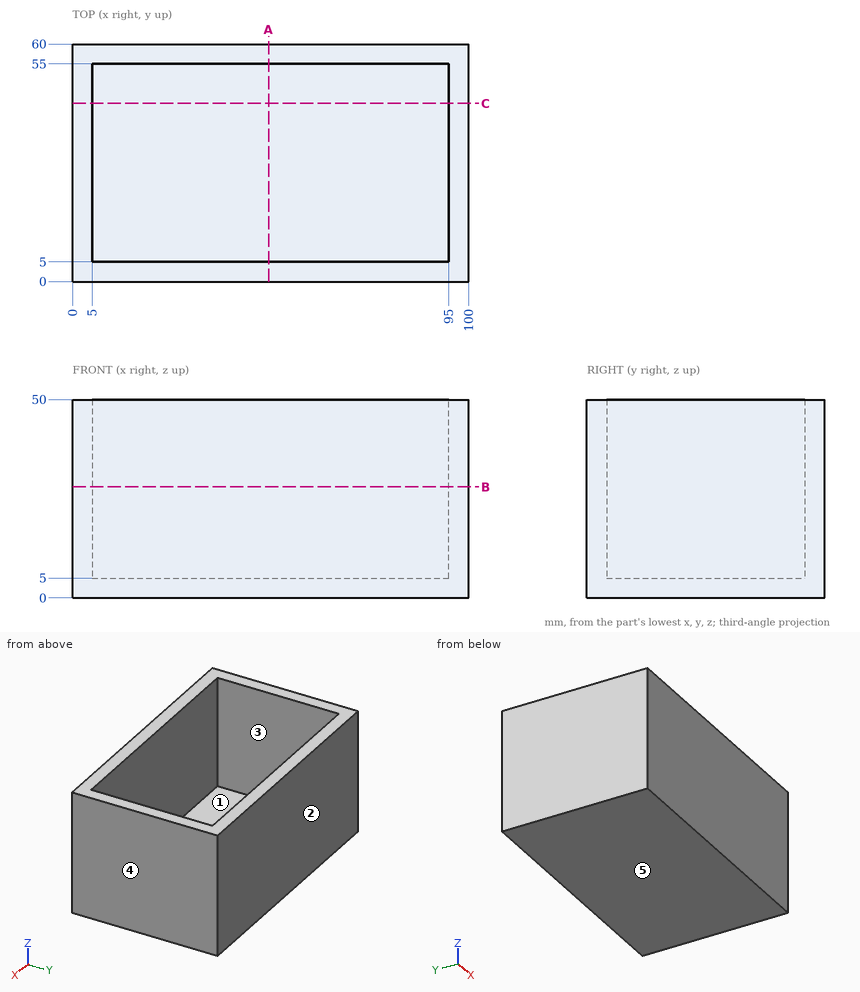
Print and shaded views of the part. All mm, measured from the part's lowest x, y and z. A direction names the side the tool comes from. Round coordinates to 2 decimals unless told otherwise and drop trailing zeros. Write each loop counter-clockwise with the first axis right and the second up, starting at its lowest first coordinate (ties: lowest second). Pieces come first, ordered by that corner, then holes.
Item 1: Cut at B-B, the plane z = 28. Give the cut face in (x, y).
Results:
outline: (0, 0) - (100, 0) - (100, 60) - (0, 60) - close; hole (5, 5) - (95, 5) - (95, 55) - (5, 55) - close
Item 2: Drop a flat-ended pin along its axis: pin 1 Ø15 at (x, y) = (50.5, 41.5) entering from +Z. Give the stop position or say it passes through.
Results:
pin 1: stops at z = 5
Item 3: Which spindle directions (+Z, -Z, +X, -X, +Y, -Y) get a long thin tool onto all of the face, cutting with end or side? Do the marked faces 1 and 2. Say none if no direction does.
Results:
face 1: +Z
face 2: +Z, -Z, +X, -X, +Y
Item 4: Cut at A-A, the plane x = 49.5. Give the cut face in (y, z).
Results:
outline: (0, 0) - (60, 0) - (60, 50) - (55, 50) - (55, 5) - (5, 5) - (5, 50) - (0, 50) - close
Item 5: Cut at C-C, the plane y = 45. Give the cut face in (x, z).
Results:
outline: (0, 0) - (100, 0) - (100, 50) - (95, 50) - (95, 5) - (5, 5) - (5, 50) - (0, 50) - close
Item 6: Two-plate mould, pull along X, no slides. Class the marked faces 3, 4 and 5: +X half, -X half, draft (parallel to the pull), parting line (faces both ways), or undercut.
Results:
face 3: undercut
face 4: +X half
face 5: draft
Item 7: Probe L1, parallel to Y at x = 83, z = 7; L2, parallel to X at y = 6.5, z = 29; L3, parallel to Z at x = 54, y = 12.5. List the from-to ranges inside material, lowest first.
Results:
L1: y = 0 to 5, 55 to 60
L2: x = 0 to 5, 95 to 100
L3: z = 0 to 5
